Design review of the part built by this model. Coordinates are the model's own, in mm. Face numbers are marked on the shaded views. A direction names the side the tool comes from. Coordinates: 2 decimals unless noted, no trailing zeros. Write each loop counter-clockwise with the first axis right and the second up, starting at its lowest first coordinate (ties: lowest second). Pieces come first, ordered by that corner, then holes.
Q1. Machinability: for the marked faces 5, 6, 7, 8 and 9, which of the approach directions +Z, -Z, +X, -X, +Y, -Y give a long, thin tool a straight path to every point of the face, cutting with its end or side? Answer none if there is none.
Q2. Insertion check: pin 1 (5 mm diameter, centred on y = -3.5, z = 3.5, fed in from +X); pin 2 (5 mm diameter, centred on y = -2.5, z = 5.5, fed in from -X); pin 3 (3 mm diameter, centred on x = 7, z = 3, fed in from +Y); pin 4 (2 mm diameter, centred on x = 51, y = -48.5, fed in from +Z). Each pin has a flat end and moves straight along its axis. Give the tip position at first contact, or say it passes through.
Q3. For probe 1 along Y at (x, z) = (7, 6); probe 2 along X at (y, z) = (-9.5, 9.25); probe 3 along Y at (x, z) = (78.5, 9.5), list the stretches that pass through material, from the lowest coordinate up.
Q4. Take a section at B-B (x = 107). Give the boundary of the cut face in (y, z), and give its area (3 significant figures).
Q5. Take a section at C-C (y = -12). Give the boundary of the cut face in (x, z).
Q6. Mouldability with a two-part tool opening along X and no side actions: class the marked faces 1, 2, 3 and 4 as pulls with the +X half, pulls with the -X half, needs draft (parallel to the pull), parting line crosses it, or undercut.
Q7. Take a section at A-A (x = 48). Give the boundary of the cut face in (y, z).
```python
from build123d import *

# Parameters (mm, degrees)
F1_DEPTH = 10.16


with BuildPart() as f1:
    # F0 (on Top) → F1 (new body)
    with BuildSketch(Plane.XY):
        Polygon((38.1, 0), (25.4, 0), (25.4, -10.16), (10.16, -10.16), (10.16, -19.05), (0, -19.05), (0, -31.75), (10.16, -31.75), (10.16, -44.45), (0, -44.45), (0, -57.15), (10.16, -57.15), (10.16, -69.85), (0, -69.85), (0, -82.55), (10.16, -82.55), (10.16, -91.44), (25.4, -91.44), (25.4, -101.6), (38.1, -101.6), (38.1, -91.44), (50.8, -91.44), (50.8, -101.6), (63.5, -101.6), (63.5, -91.44), (76.2, -91.44), (76.2, -101.6), (88.9, -101.6), (88.9, -91.44), (104.14, -91.44), (104.14, -82.55), (114.3, -82.55), (114.3, -69.85), (104.14, -69.85), (104.14, -57.15), (114.3, -57.15), (114.3, -44.45), (104.14, -44.45), (104.14, -31.75), (114.3, -31.75), (114.3, -19.05), (104.14, -19.05), (104.14, -10.16), (88.9, -10.16), (88.9, 0), (76.2, 0), (76.2, -10.16), (63.5, -10.16), (63.5, 0), (50.8, 0), (50.8, -10.16), (38.1, -10.16), align=None)
        with BuildLine():
            ThreePointArc((22.225, -53.34), (24.084872, -48.849872), (28.575, -46.99))
            Line((28.575, -46.99), (85.725, -46.99))
            ThreePointArc((85.725, -46.99), (90.215128, -48.849872), (92.075, -53.34))
            ThreePointArc((92.075, -53.34), (90.215128, -57.830128), (85.725, -59.69))
            Line((85.725, -59.69), (28.575, -59.69))
            ThreePointArc((28.575, -59.69), (24.084872, -57.830128), (22.225, -53.34))
        make_face(mode=Mode.SUBTRACT)
    extrude(amount=F1_DEPTH)


solid = f1.part
```
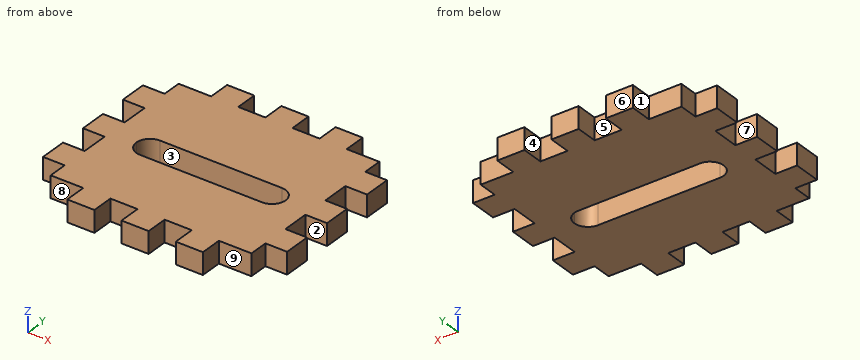
Response:
1. face 5: +Z, -Z, +Y
1. face 6: +Z, -Z, +X, -X, +Y
1. face 7: +Z, -Z, -X
1. face 8: +Z, -Z, -X, -Y
1. face 9: +Z, -Z, +X, -Y
2. pin 1: stops at x = 88.9
2. pin 2: stops at x = 25.4
2. pin 3: stops at y = -19.05
2. pin 4: passes through
3. probe 1: y = -82.55 to -69.85, -57.15 to -44.45, -31.75 to -19.05
3. probe 2: x = 25.4 to 38.1, 50.8 to 63.5, 76.2 to 88.9
3. probe 3: y = -101.6 to -59.69, -46.99 to 0
4. outline: (-82.55, 0) - (-69.85, 0) - (-69.85, 10.16) - (-82.55, 10.16) - close; (-57.15, 0) - (-44.45, 0) - (-44.45, 10.16) - (-57.15, 10.16) - close; (-31.75, 0) - (-19.05, 0) - (-19.05, 10.16) - (-31.75, 10.16) - close
4. area: 387 mm2
5. outline: (10.16, 0) - (104.14, 0) - (104.14, 10.16) - (10.16, 10.16) - close
6. face 1: pulls with the -X half
6. face 2: needs draft
6. face 3: undercut
6. face 4: undercut
7. outline: (-91.44, 0) - (-59.69, 0) - (-59.69, 10.16) - (-91.44, 10.16) - close; (-46.99, 0) - (-10.16, 0) - (-10.16, 10.16) - (-46.99, 10.16) - close
